Read the model definition and answer for the solid it produces. Units are mm, in the model's axes. Coordinates: 2 decimals unless noted, no trailing zeros. Write each loop counter-clockwise with the first axis right and the second up, starting at its lowest first coordinate (ties: lowest second). Pieces come first, ordered by that corner, then holes.
(1) Section B-B on z = 16.5 is taken. Write down the section's boundary in (x, y).
(2) Given pin 1 (12 mm diameter, centred on y = -3.5, z = 15, fed in from -X); pin 2 (1.4 mm diameter, centred on x = -113, y = -39, fed in from -Z), each flat-ended and moving along its own axis, determine where each tip first touches the part or whether it passes through.
(3) Section A-A on y = 21 is taken. Write down the section's boundary in (x, z), then the cut area to 3 significant figures.
(4) Find the intervals of material crossed by probe 1 along X at (y, z) = (-20.5, 8); probe 2 along X at (y, z) = (29.5, -4), in increasing order.
from build123d import *

# Parameters (mm, degrees)
F0_W     = 254
F0_H     = 127
F1_DEPTH = 15.9
F3_DEPTH = 127
F4_W     = 4.5899346401
F4_H     = 127
F4_W_2   = 249.4100653599
F5_DEPTH = 19.05
F7_DEPTH = 127


# Not quite as in the source:
# - the program builds the solid bodies; features that only make, move or delete a surface that nothing else refers to are left out


with BuildPart() as f1:
    # F0 (on Top) → F1 (new body)
    with BuildSketch(Plane.XY):
        with Locations((10.4389302433, -20.9855538282)):
            Rectangle(F0_W, F0_H)
    extrude(amount=-F1_DEPTH)

    # F2 (on face) → F3 (cut)
    with BuildSketch(Plane.XZ.offset(84.4855538282)):
        Polygon((-116.5610697567, 0), (-116.5610697567, -7.95), (-111.9711351167, 0), align=None)
        Polygon((-111.9711351167, -15.9), (-116.5610697567, -7.95), (-116.5610697567, -15.9), align=None)
    extrude(amount=-F3_DEPTH, mode=Mode.SUBTRACT)

    # F4 (on face) → F5 (join)
    with BuildSketch(Plane.XY):
        with Locations((-114.2661024367, -20.9855538282)):
            Rectangle(F4_W, F4_H)
        with Locations((12.7338975633, -20.9855538282)):
            Rectangle(F4_W_2, F4_H)
    extrude(amount=F5_DEPTH)

    # F6 (on face) → F7 (cut)
    with BuildSketch(Plane.XZ.offset(84.4855538282)):
        Polygon((-116.5610697567, 19.05), (-116.5610697567, 0), (-105.5625471287, 19.05), align=None)
    extrude(amount=-F7_DEPTH, mode=Mode.SUBTRACT)


solid = f1.part
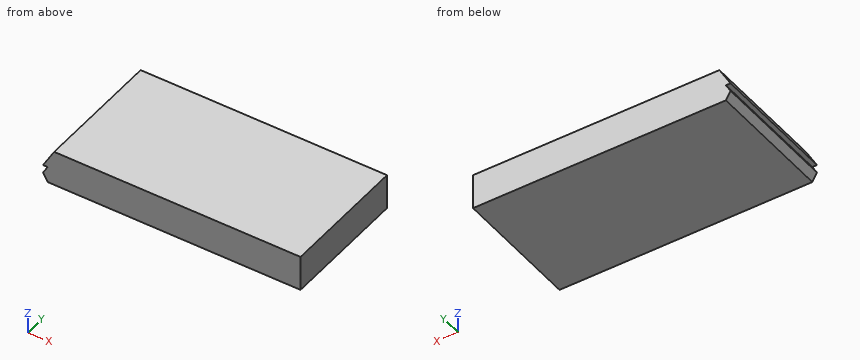
Response:
1. outline: (-107.03, -84.49) - (137.44, -84.49) - (137.44, 42.51) - (-107.03, 42.51) - close
2. pin 1: stops at x = -111.36
2. pin 2: stops at z = -15.33
3. outline: (-116.56, -7.95) - (-111.97, -15.9) - (137.44, -15.9) - (137.44, 19.05) - (-105.56, 19.05) - (-116.56, 0) - (-111.97, 0) - close
3. area: 8,740 mm2
4. probe 1: x = -111.94 to 137.44
4. probe 2: x = -114.28 to 137.44
